Verification items for the finished model (mm, model axes). A direction names the side the tool comes from. Give positions to 0.01 mm unless a question says otherwise; leave off trailing zeros. Loops run counter-clockwise (first coordinate to the right, second up) from the corner with the lowest first, then second, coordinate; pieces in that order, holes last. Notation, with made-up numbers: M 44,-13 L 59,-13 A21 ccw 59,3 Z; hole C 3,74.25 d5. An arc over 180 degrees is marked long. Use a Markdown table: item, result.
from build123d import *

# Parameters (mm, degrees)
SKETCH1_R           = 1.75
BOSS_EXTRUDE1_DEPTH = 2.2


with BuildPart() as part:
    # Sketch1 → Boss-Extrude1 (new body)
    with BuildSketch(Plane(origin=(0, 0, 0), x_dir=(1, 0, 0), z_dir=(0, 1, 0))):
        with BuildLine():
            Line((-32.452490814, -50.090677738), (-34.898824615, -52.53701154))
            Line((-34.898824615, -52.53701154), (-58.615441718, -76.253628642))
            ThreePointArc((-58.615441718, -76.253628642), (-59.494121374, -78.374948986), (-58.615441718, -80.496269329))
            Line((-58.615441718, -80.496269329), (-56.546018533, -82.565692514))
            Line((-56.546018533, -82.565692514), (-58.313785486, -84.333459467))
            Line((-58.313785486, -84.333459467), (-51.897927296, -90.749317656))
            Line((-51.897927296, -90.749317656), (-53.453562215, -92.304952575))
            Line((-53.453562215, -92.304952575), (-59.869420404, -85.889094386))
            Line((-59.869420404, -85.889094386), (-61.849319392, -87.868993373))
            Line((-61.849319392, -87.868993373), (-55.433461202, -94.284851562))
            Line((-55.433461202, -94.284851562), (-48.36239339, -101.355919374))
            Line((-48.36239339, -101.355919374), (-41.946535201, -107.771777564))
            Line((-41.946535201, -107.771777564), (-39.966636214, -105.791878576))
            Line((-39.966636214, -105.791878576), (-46.382494403, -99.376020387))
            Line((-46.382494403, -99.376020387), (-44.826859485, -97.820385468))
            Line((-44.826859485, -97.820385468), (-38.411001295, -104.236243658))
            Line((-38.411001295, -104.236243658), (-36.643234342, -102.468476705))
            Line((-36.643234342, -102.468476705), (-34.573811157, -104.53789989))
            ThreePointArc((-34.573811157, -104.53789989), (-32.452490814, -105.416579546), (-30.33117047, -104.53789989))
            Line((-30.33117047, -104.53789989), (-6.614553368, -80.821282787))
            Line((-6.614553368, -80.821282787), (-4.168219566, -78.374948986))
            Line((-4.168219566, -78.374948986), (-6.237642751, -76.305525801))
            ThreePointArc((-6.237642751, -76.305525801), (-7.116322408, -74.184205457), (-6.237642751, -72.062885114))
            Line((-6.237642751, -72.062885114), (-4.469875798, -70.295118161))
            Line((-4.469875798, -70.295118161), (-10.833836829, -63.93115713))
            Line((-10.833836829, -63.93115713), (-9.419623267, -62.516943568))
            Line((-9.419623267, -62.516943568), (-16.594485396, -55.342081438))
            Line((-16.594485396, -55.342081438), (-18.008698958, -56.756295001))
            Line((-18.008698958, -56.756295001), (-24.372659989, -50.39233397))
            Line((-24.372659989, -50.39233397), (-26.140426942, -52.160100923))
            ThreePointArc((-26.140426942, -52.160100923), (-28.261747285, -53.03878058), (-30.383067629, -52.160100923))
            Line((-30.383067629, -52.160100923), (-32.452490814, -50.090677738))
        make_face()
        with Locations(Location((-32.452490814, -99.588152421, 0), (0, 0, 270))):
            Circle(SKETCH1_R, mode=Mode.SUBTRACT)
        with Locations(Location((-53.665694249, -78.374948986, 0), (0, 0, 270))):
            Circle(SKETCH1_R, mode=Mode.SUBTRACT)
        with Locations(Location((-11.239287378, -78.374948986, 0), (0, 0, 270))):
            Circle(SKETCH1_R, mode=Mode.SUBTRACT)
        with Locations(Location((-32.452490814, -57.16174555, 0), (0, 0, 270))):
            Circle(SKETCH1_R, mode=Mode.SUBTRACT)
    extrude(amount=BOSS_EXTRUDE1_DEPTH)


solid = part.part
(1) Cross-section at D-D on y = 0.85. State how many separate pieces and enclosed holes the cut face has, then the cut area to 3 significant figures.
Results below:
| item | result |
|---|---|
| separate pieces | 1 |
| enclosed holes | 4 |
| area | 1,910 mm^2 |
(2) Cross-section at A-A on z = 58. Record the cut outline in (x, y), then the cut area to 3 significant figures.
Results below:
| item | result |
|---|---|
| outline | M -40.36,0 L -33.99,0 L -33.99,2.2 L -40.36,2.2 Z; M -30.92,0 L -13.94,0 L -13.94,2.2 L -30.92,2.2 Z |
| area | 51.4 mm^2 |
(3) Set-up check for faces 4 (the flat face through (-57.42, 1.08, 83.44)), 5 (the flat face through (-5.188, 1.085, 77.355)), 6 (the flat face through (-56.62, 1.08, 89.14)): record each of +Z, -Z, +X, -X, +Y, -Y from which the full face is reachable in a straight line by a thin tool's end or side.
Results below:
| item | result |
|---|---|
| face 4 | -X, +Y, -Y |
| face 5 | +X, +Y, -Y |
| face 6 | +Y, -Y |
(4) Gauge pin test, flat end, axial feed: P1, Ø1, axis at y = 0.5, z = 57.5, coming from the -X side. Record the tip position at first contact, or that the pin passes through.
Results below:
| item | result |
|---|---|
| P1 | x = -40.36 |
(5) Material ranges on line 1 (Z direction, x = -57.5, y = 1.3); line 2 (X direction, y = 2.05, z = 100); line 3 (X direction, y = 1.4, z = 79), recorded low to high.
Results below:
| item | result |
|---|---|
| line 1 | 75.14 to 81.61, 83.52 to 85.15, 88.26 to 92.22 |
| line 2 | -49.72 to -45.76, -42.65 to -34.15, -30.75 to -25.79 |
| line 3 | -59.43 to -55.3, -52.03 to -12.87, -9.6 to -4.79 |
(6) Draft check along X on faces 1 (the flat face through (-10.1, 1.1, 63.2)), 2 (the flat face through (-55.15, 1.08, 87.5)), 3 (the flat face through (-60.85, 1.08, 86.87)). Enter one of: +X half, -X half, draft (parallel to the pull), parting line (faces both ways), or undercut.
Results below:
| item | result |
|---|---|
| face 1 | +X half |
| face 2 | undercut |
| face 3 | -X half |
(7) Cross-section at B-B on z = 91.5. Record the cut outline in (x, y), then the cut area to 3 significant figures.
Results below:
| item | result |
|---|---|
| outline | M -58.22,0 L -54.26,0 L -54.26,2.2 L -58.22,2.2 Z; M -52.65,0 L -17.29,0 L -17.29,2.2 L -52.65,2.2 Z |
| area | 86.5 mm^2 |
(8) Cross-section at C-C on x = -29.5. Record the cut outline in (y, z), then the cut area to 3 significant figures.
Results below:
| item | result |
|---|---|
| outline | M 0,52.77 L 2.2,52.77 L 2.2,103.71 L 0,103.71 Z |
| area | 112 mm^2 |
